Geometry: final body of the model. Coordinates: model frame, mm. Round coordinates to 2 decimals unless told otherwise and drop trailing zeros. Loops run counter-clockwise (first coordinate to the right, second up) from the corner with the lowest first, then second, coordinate; pieces in that order, holes last. Notation, with made-up numbers: M -28,24.5 L 9,24.5 A15 cw 9,34.5 Z; hole C 43.5,49.25 d4. An arc over 180 degrees is marked long. Answer as a JSON object with one key per item and string values.
from build123d import *

# Parameters (mm, degrees)
SKETCH_1_W                   = 40
SKETCH_1_H                   = 5.3
EXTRUDE_1_DEPTH              = 4
CUT_EXTRUDE_1_DEPTH          = 41.547379693
SKETCH_3_R                   = 1.5
CUT_EXTRUDE_2_DEPTH          = 41.547379693
HOLE_WIZARD_M3_1_D           = 3.4
HOLE_WIZARD_M3_1_CSINK_D     = 6.72
HOLE_WIZARD_M3_1_CSINK_ANGLE = 90


with BuildPart() as part:
    # 草图1 → 凸台-拉伸1 (new body)
    with BuildSketch(Plane.XY):
        with Locations((20, 2.65)):
            Rectangle(SKETCH_1_W, SKETCH_1_H)
    extrude(amount=EXTRUDE_1_DEPTH)

    # 草图2 → 切除-拉伸1 (cut, through all)
    with BuildSketch(Plane(origin=(40, 0, 0), x_dir=(0, 0, -1), z_dir=(1, 0, 0))):
        Polygon((-4, 5.3), (0, 5.3), (0, 4.8), align=None)
    extrude(amount=-CUT_EXTRUDE_1_DEPTH, mode=Mode.SUBTRACT)

    # 草图3 → 切除-拉伸2 (cut, through all)
    with BuildSketch(Plane.XY.offset(4)):
        with Locations((12, 2.5)):
            Circle(SKETCH_3_R)
        with Locations(Location((28, 2.5, 0), (0, 0, 180))):
            Circle(SKETCH_3_R)
    extrude(amount=-CUT_EXTRUDE_2_DEPTH, mode=Mode.SUBTRACT)

    # M3 六角凹锥坑螺钉的锥形沉头孔1 (through all)
    with Locations(Plane(origin=(12, 2.5, 4), x_dir=(1, 0, 0), z_dir=(0, 0, 1))):
        with Locations((0, 0), (16, 0)):
            CounterSinkHole(HOLE_WIZARD_M3_1_D / 2, HOLE_WIZARD_M3_1_CSINK_D / 2, counter_sink_angle=HOLE_WIZARD_M3_1_CSINK_ANGLE)


solid = part.part
1) Section query A-A (y = 2.5). Return the cut outline in (x, z).
Results:
{"outline": "M 0,0 L 10.3,0 L 10.3,2.34 L 8.64,4 L 0,4 Z; M 13.7,0 L 26.3,0 L 26.3,2.34 L 24.64,4 L 15.36,4 L 13.7,2.34 Z; M 29.7,0 L 40,0 L 40,4 L 31.36,4 L 29.7,2.34 Z"}
2) Pin query (flat end, axial travel): P1, Ø2, axis at y = 4.5, z = 3.5, coming from the -X side. Return the tip coordinate at first contact, or that it passes through.
Results:
{"P1": "x = 0"}
3) Section query D-D (z = 0.4). Return the cut outline in (x, y), and give its area (3 significant figures).
Results:
{"outline": "M 0,0 L 40,0 L 40,4.85 L 0,4.85 Z; hole C 12,2.5 d3.4; hole C 28,2.5 d3.4", "area": "176 mm2"}
4) Section query B-B (x = 12). Return the cut outline in (y, z), and give its area (3 significant figures).
Results:
{"outline": "M 0,0 L 0.8,0 L 0.8,2.34 L 0,3.14 Z; M 4.2,0 L 4.8,0 L 5.22,3.36 L 4.2,2.34 Z", "area": "4.39 mm2"}
5) Section query C-C (z = 3.5). Return the cut outline in (x, y).
Results:
{"outline": "M 0,0 L 10.61,0 A2.86 cw 11.17,5.24 L 0,5.24 Z; M 12.83,5.24 A2.86 cw 13.39,0 L 26.61,0 A2.86 cw 27.17,5.24 Z; M 28.83,5.24 A2.86 cw 29.39,0 L 40,0 L 40,5.24 Z"}
6) Ray query, line 1 (X direction, y = 2.5, z = 0.95); line 2 (X direction, y = 4.35, z = 2.9); line 3 (Y direction, x = 28, z = 1.25). Return the intervals inside material, ascending.
Results:
{"line 1": "0 to 10.3, 13.7 to 26.3, 29.7 to 40", "line 2": "0 to 10.7, 13.3 to 26.7, 29.3 to 40", "line 3": "0 to 0.8, 4.2 to 4.96"}
7) Pull-direction query (X, two-part tool) for faces 1 (the cylindrical face through (10.38, 3.01, 1.15)), 2 (the flat face through (40, 3, 2)), 3 (the flat face through (20.28, 5.046, 1.972)); classes: +X half, -X half, draft (parallel to the pull), parting line (faces both ways), or undercut.
Results:
{"face 1": "undercut", "face 2": "+X half", "face 3": "draft"}
